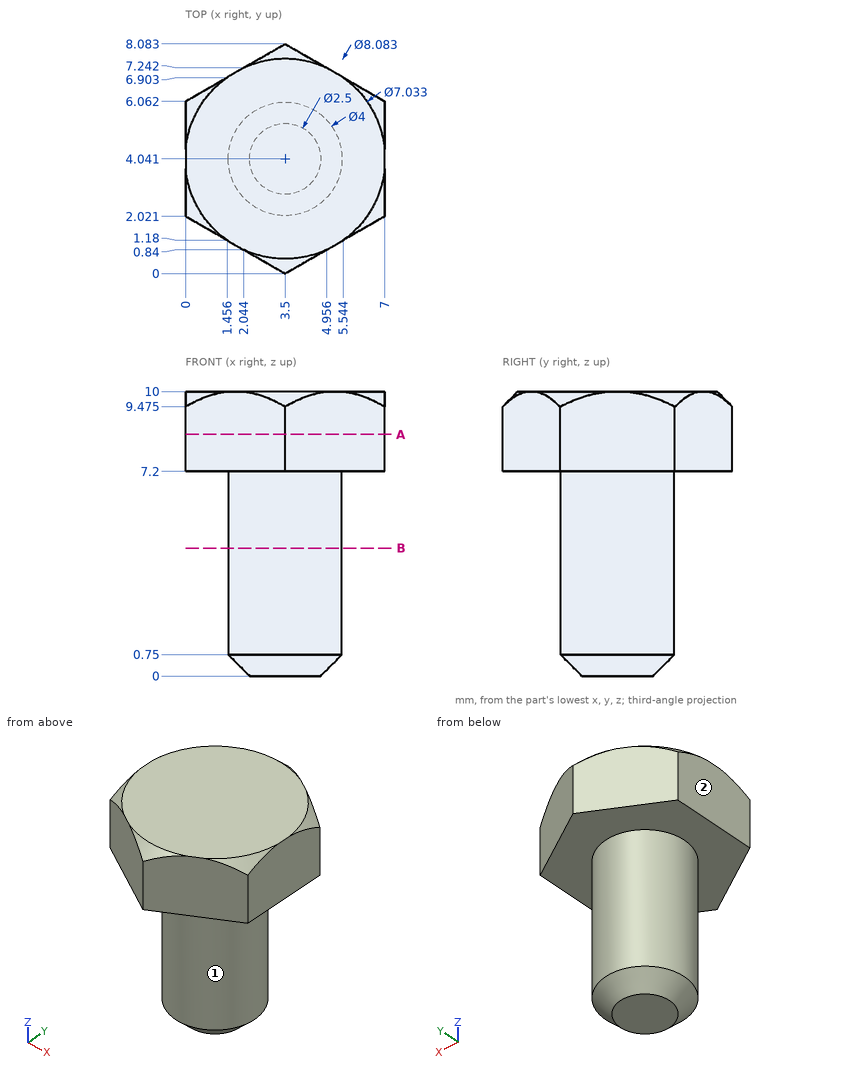
The drawing under review shows one solid part. Ordinate dimensions are in mm from its lowest x, y, z. A direction names the side the tool comes from. Give positions to 0.01 mm unless a question says otherwise; leave off trailing zeros. Order: outer loops, then holes, each group sorted by start corner. A loop starts at its lowest first (then second) coordinate and runs counter-clockwise, first axis right, second up. Notation, with made-up numbers: (42.5, 77) - (64.5, 77) arc R24 ccw to (64.5, 99) - close; hole circle Ø2 at (-33.75, 0.5). An arc over 180 degrees is marked (long way). Answer as a JSON object with one key per item and string values. Group by question number.
Item 1: Take a section at A-A on z = 8.5. Give the boundary of the cut face in (x, y).
Item 2: Take a section at B-B on z = 4.5. Give the boundary of the cut face in (x, y).
Item 3: Clearance check with flat-ended pins moving along their axes: pin 1 Ø4 at (x, z) = (5, 3) entering from -Y; pin 2 Ø2 at (x, z) = (5.5, 8.5) entering from -Y; pin 3 Ø3 at (x, z) = (1.5, 5) entering from -Y (1 decimal). State where each tip first meets the part, or that it passes through.
Item 4: Wall thickness on line 1 along Z through (x, y) = (3, 6.5); line 2 along X through (y, z) = (4, 4.25); line 3 along X through (y, z) = (5.5, 2.25): over which ranges is each line inside the solid? List them lowest first.
Item 5: Machinability: for the marked faces 1 and 2, which of the approach directions +Z, -Z, +X, -X, +Y, -Y give a long, thin tool a straight path to every point of the face, cutting with its end or side? Answer none if there is none.
Reported:
{
 "1": {"outline": "(0, 2.02) - (3.5, 0) - (7, 2.02) - (7, 6.06) - (3.5, 8.08) - (0, 6.06) - close"},
 "2": {"outline": "circle Ø4 at (3.5, 4.04)"},
 "3": {"pin 1": "y = 2.04", "pin 2": "y = 0.58", "pin 3": "y = 2.1"},
 "4": {"line 1": "7.2 to 10", "line 2": "1.5 to 5.5", "line 3": "2.13 to 4.87"},
 "5": {"face 1": "-Z", "face 2": "+Z, -Z, -X, +Y, -Y"}
}
